The listing builds one solid part. Answer for the finished solid, in the listing's coordinates (mm). Coordinates: 2 decimals unless noted, no trailing zeros. Write each loop counter-clockwise with the first axis right and the second up, starting at its lowest first coordinate (ties: lowest second). Pieces come first, ordered by that corner, then holes.
(1) The part is cut by section D-D on y = 27. Determine the outline of the cut face in (x, z).
(2) The part is cut by section A-A on y = 55. Determine the outline of the cut face in (x, z), plus the area to 3 significant figures.
(3) The part is cut by section B-B on x = 0.95. Give the number of separate pieces and of enclosed holes in the cut face, plus the area to 3 significant figures.
(4) Given P1, Ø8.5, axis at y = 35.81, z = 69.4, coming from the +X side; P2, Ø3, axis at y = -40.39, z = -57.6, coming from the -X side, each flat-ended and moving along its own axis, determine where each tip first touches the part or whether it passes through.
(5) Straight lines are drawn through the part: line 1 (Y direction, x = 2.5, z = -6); line 2 (Y direction, x = 2.3, z = 0); line 3 (Y direction, x = 1.65, z = 35.5). For each, find the intervals that lie inside material, in ascending order.
(6) The part is cut by section C-C on z = 99. Determine the outline of the cut face in (x, y), plus the area to 3 significant figures.
Autodesk Inventor part; units mm, degrees
ref_plane "YZ Plane" through (0, 0, 0) normal (1, 0, 0) x (0, 1, 0)
ref_plane "XZ Plane" through (0, 0, 0) normal (0, 1, 0) x (-1, 0, 0)
ref_plane "XY Plane" through (0, 0, 0) normal (0, 0, 1) x (1, 0, 0)
sketch "Sketch1" plane through (0, 0, 0) normal (1, 0, 0) x (0, 1, 0)
  line L0 (23.1056, 132.8959) -> (-53.0944, 132.8959)
  line L1 (-53.0944, 132.8959) -> (-53.0944, -121.1041)
  line L2 (-53.0944, -121.1041) -> (23.1056, -121.1041)
  line L3 (23.1056, 132.8959) -> (73.9056, 5.8959)
  line L4 (73.9056, 5.8959) -> (23.1056, -121.1041)
  line L5 (73.9056, 5.8959) -> (-53.0944, 5.8959) construction
  point P0 (0, 0)
  dimension "d0" = 76.2
  dimension "d1" = 254
extrude "Extrusion1" add sketch "Sketch1" along normal blind 2.9972
sketch "Sketch2" plane through (2.9972, 0, 0) normal (1, 0, 0) x (0, 0, -1)
  circle A0 centre (-120.1959, -40.3944) radius 1.7272
  line L0 (-132.8959, 23.1056) -> (-132.8959, -53.0944)
  line L1 (-132.8959, -53.0944) -> (121.1041, -53.0944)
  point P0 (0, 0)
  dimension "d5" = 12.7
  dimension "d6" = 12.7
  dimension "d7" = 3.4544
extrude "Extrusion2" cut sketch "Sketch2" against normal through all
pattern_linear "Rectangular Pattern1" count 10 spacing 25.4 along (0, 0, -1) of "Extrusion2"
sketch "Sketch3" plane through (2.9972, 0, 0) normal (1, 0, 0) x (0, 0, -1)
  circle A0 centre (-5.8959, 48.5056) radius 14.2875
  line L0 (121.1041, 23.1056) -> (-5.8959, 73.9056)
  line L1 (-5.8959, 73.9056) -> (-5.8959, 48.5056) construction
  point P0 (0, 0)
  dimension "d13" = 28.575
  dimension "d14" = 25.4
extrude "Extrusion3" cut sketch "Sketch3" against normal through all
sketch "Sketch4" plane through (2.9972, 0, 0) normal (1, 0, 0) x (0, 0, -1)
  circle A0 centre (-69.3959, 35.8056) radius 3.175
  circle A1 centre (57.6041, 35.8056) radius 3.175
  line L0 (-69.3959, 35.8056) -> (57.6041, 35.8056) construction
  line L1 (121.1041, 23.1056) -> (-5.8959, 73.9056)
  line L2 (-5.8959, 73.9056) -> (-5.8959, 17.32) construction
  point P0 (0, 0)
  dimension "d17" = 6.35
  dimension "d18" = 127
  dimension "d19" = 63.5
  dimension "d20" = 38.1
extrude "Extrusion4" cut sketch "Sketch4" against normal through all
fillet "Fillet1" radius 19.05 1 edges at (1.4986, 73.9056, 5.8959)
properties part number "Jeep Plate" material "Polycarbonate, Clear"
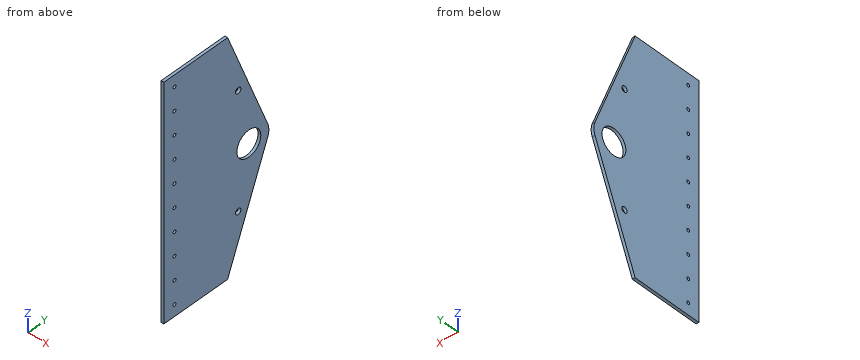
Model answer:
1. outline: (0, -111.37) - (3, -111.37) - (3, 123.16) - (0, 123.16) - close
2. outline: (0, -41.37) - (3, -41.37) - (3, -6.83) - (0, -6.83) - close; (0, 18.62) - (3, 18.62) - (3, 53.16) - (0, 53.16) - close
2. area: 207 mm2
3. separate pieces: 1
3. enclosed holes: 13
3. area: 25,000 mm2
4. P1: stops at x = 3
4. P2: passes through
5. line 1: y = -53.09 to -41.92, -38.87 to 40.59, 56.42 to 69.15
5. line 2: y = -53.09 to 35.49, 61.52 to 71.5
5. line 3: y = -53.09 to 62.06
6. outline: (0, -53.09) - (3, -53.09) - (3, 36.66) - (0, 36.66) - close
6. area: 269 mm2
